CAD build for the part. Positions are in the model's coordinates, mm. Face numbers are marked on the shaded views. A direction names the side the tool comes from. Round coordinates to 2 decimals unless told otherwise and drop trailing zeros. Loops run counter-clockwise (first coordinate to the right, second up) from the corner with the lowest first, then second, coordinate; pieces in that order, holes last. Notation, with made-up numbers: M 78.25,56.25 L 100.25,56.25 A27 cw 100.25,93.25 Z; hole C -32.5,-38.75 d2. An arc over 180 degrees is marked long. Use one line per item in the form item = value.
from build123d import *

# Parameters (mm, degrees)
SKETCH_1_R               = 15
SKETCH_1_R_2             = 11.75
EXTRUDE_1_DEPTH          = 4
SKETCH_2_R               = 11.75
SKETCH_2_R_2             = 9.75
EXTRUDE_2_DEPTH          = 1
FILLET_1_R               = 1
FILLET_2_R               = 1
SKETCH_3_R               = 17.5
SKETCH_3_R_2             = 11.75
EXTRUDE_3_DEPTH          = 0.9
CUT_EXTRUDE_1_DEPTH      = 27.009613607
FILLET_3_R               = 2
FILLET_4_R               = 1
SKETCH_6_R               = 1
CUT_EXTRUDE_2_DEPTH      = 6.5
PATTERN_CIRCULAR_2_COUNT = 3
FILLET_6_R               = 0.5
CHAMFER_1_SIZE           = 0.4
CHAMFER_1_SIZE2          = 2


# Some blends are built 0.0001 mm under size
with BuildPart() as part:
    # 草图1 → 凸台-拉伸1 (new, symmetric)
    with BuildSketch(Plane.XY):
        Circle(SKETCH_1_R)
        Circle(SKETCH_1_R_2, mode=Mode.SUBTRACT)
    extrude(amount=EXTRUDE_1_DEPTH, both=True)

    # 草图2 → 凸台-拉伸2 (add)
    with BuildSketch(Plane(origin=(0, 0, -4), x_dir=(-1, 0, 0), z_dir=(0, 0, -1))):
        Circle(SKETCH_2_R)
        Circle(SKETCH_2_R_2, mode=Mode.SUBTRACT)
    extrude(amount=-EXTRUDE_2_DEPTH)

    # 圆角1
    fillet_1_edges = [part.edges().sort_by_distance(p)[0] for p in [
        (-15, 0, -4),
    ]]
    fillet(fillet_1_edges, radius=FILLET_1_R)

    # 圆角2
    fillet_2_edges = [part.edges().sort_by_distance(p)[0] for p in [
        (9.75, 0, -4),
    ]]
    fillet(fillet_2_edges, radius=FILLET_2_R - 0.0001)  # a hair under: the kernel refuses the full size

    # 草图3 → 凸台-拉伸3 (add)
    with BuildSketch(Plane.XY.offset(4)):
        Circle(SKETCH_3_R)
        with Locations(Location((0, 0, 0), (0, 0, 180))):
            Circle(SKETCH_3_R_2, mode=Mode.SUBTRACT)
    extrude(amount=EXTRUDE_3_DEPTH)

    # 草图4 → 切除-拉伸1 (cut, through all)
    with BuildSketch(Plane(origin=(0, 0, 4), x_dir=(-1, 0, 0), z_dir=(0, 0, -1))):
        with BuildLine():
            Line((-20.056660766, 2), (-15.067846561, 2))
            ThreePointArc((-15.067846561, 2), (-15.2, 0), (-15.067846561, -2))
            Line((-15.067846561, -2), (-20.056660766, -2))
            Line((-20.056660766, -2), (-20.056660766, 2))
        make_face()
    cut_extrude_1 = extrude(amount=-CUT_EXTRUDE_1_DEPTH, mode=Mode.SUBTRACT)

    # 镜向1: 切除-拉伸1 across plane
    add(cut_extrude_1.mirror(Plane(origin=(0, 0, 0), x_dir=(0, 0, 1), z_dir=(1, 0, 0))), mode=Mode.SUBTRACT)

    # 圆角3
    fillet_3_edges = [part.edges().sort_by_distance(p)[0] for p in [
        (-15.067846561, -2, 4.45),
        (-15.067846561, 2, 4.45),
        (15.067846561, -2, 4.45),
        (15.067846561, 2, 4.45),
    ]]
    fillet(fillet_3_edges, radius=FILLET_3_R - 0.0001)  # a hair under: the kernel refuses the full size

    # 圆角4
    fillet_4_edges = [part.edges().sort_by_distance(p)[0] for p in [
        (17.385338651, 2, 4.45),
        (17.385338651, -2, 4.45),
        (-17.385338651, -2, 4.45),
        (-17.385338651, 2, 4.45),
    ]]
    fillet(fillet_4_edges, radius=FILLET_4_R)

    # 草图6 → 切除-拉伸2 (cut)
    with BuildSketch(Plane.XY.offset(4.9)):
        with Locations((0, 14.3)):
            Circle(SKETCH_6_R)
    cut_extrude_2 = extrude(amount=-CUT_EXTRUDE_2_DEPTH, mode=Mode.SUBTRACT)

    # 阵列(圆周)2: 切除-拉伸2 ×3 about axis
    pattern_circular_2_axis = Axis((0, 0, 0), (0, 0, 1))
    for i in range(1, PATTERN_CIRCULAR_2_COUNT):
        add(cut_extrude_2.rotate(pattern_circular_2_axis, i * 360 / PATTERN_CIRCULAR_2_COUNT), mode=Mode.SUBTRACT)

    # 圆角6
    # the kernel refuses this fillet: 0.5 mm, written as the material it takes off along each edge
    with BuildSketch(Plane(origin=(-0.73119563, 14.982167832, -1.6), x_dir=(-0.997111465428935, -0.07595212643607639, 0), z_dir=(0, 0, 1)), Plane(origin=(13.340535761, -6.857849926, -1.6), x_dir=(0.4327792617493751, 0.9014999226842262, 0), z_dir=(0, 0, 1)), Plane(origin=(-12.609340132, -8.124317906, -1.6), x_dir=(0.5643322036795584, -0.8255477962481478, 0), z_dir=(0, 0, 1))) as fillet_6_piece_1:
        with BuildLine():
            CenterArc((0.804059787, 0.49981424), FILLET_6_R, 170.950986261, 100.610876057)
            ThreePointArc((0.310282709, 0.578453903), (0.203956844, 0.26304232), (0, 0))
            ThreePointArc((0, 0), (0.40884396, -0.005572815), (0.817687919, 0))
        make_face()
    extrude(amount=5.6, mode=Mode.SUBTRACT)
    with BuildSketch(Plane(origin=(0.73119563, 14.982167832, -1.6), x_dir=(0.997111465428935, -0.07595212643607635, 0), z_dir=(0, 0, 1)), Plane(origin=(12.609340132, -8.124317906, -1.6), x_dir=(-0.5643322036795624, -0.825547796248145, 0), z_dir=(0, 0, 1)), Plane(origin=(-13.340535761, -6.857849926, -1.6), x_dir=(-0.4327792617493753, 0.9014999226842261, 0), z_dir=(0, 0, 1))) as fillet_6_piece_2:
        with BuildLine():
            CenterArc((0.804059787, -0.49981424), FILLET_6_R, 88.438137682, 100.610876057)
            ThreePointArc((0.310282709, -0.578453903), (0.203956844, -0.26304232), (0, 0))
            ThreePointArc((0, 0), (0.40884396, 0.005572815), (0.817687919, 0))
        make_face()
    extrude(amount=5.6, mode=Mode.SUBTRACT)

    # 倒角1
    chamfer_1_edges = [part.edges().sort_by_distance(p)[0] for p in [
        (11.75, 0, 4.9),
    ]]
    chamfer_1_side = [part.faces().sort_by_distance(p)[0] for p in [
        (15.179125182, 1.457318687, 4.9),
    ]]
    chamfer(chamfer_1_edges, length=CHAMFER_1_SIZE, length2=CHAMFER_1_SIZE2, reference=chamfer_1_side[0])


solid = part.part
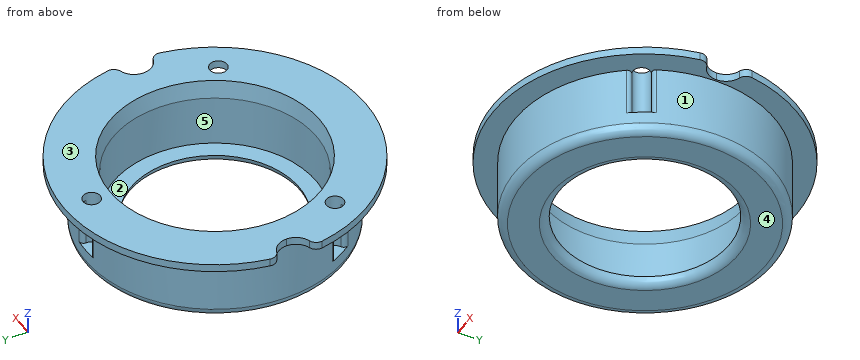
1. Pull direction X, two halves, no side cores. Call the marked faces 1, 2 and 3: +X half, -X half, draft (parallel to the pull), parting line (faces both ways), or undercut.
Completed:
face_1 = parting line
face_2 = undercut
face_3 = draft
2. Cut at A-A on x = 0. State how many separate pieces and enclosed holes the cut face has, and give its area (3 significant figures).
Completed:
separate_pieces = 3
enclosed_holes = 0
area = 53.4 mm2
3. Probe line 1 along Y through (x, z) = (0, 1); line 2 along X through (y, z) = (-0.5, -1.5); line 3 along X through (y, z) = (-8, -2). List the from-to ranges inside material, lowest first. Write a range as from..to.
Completed:
line_1 = -15..-11.75, 11.75..13.3
line_2 = -14.99..-11.74, 11.74..14.99
line_3 = -12.69..-8.61, 8.61..12.69
4. Cut at D-D on z = -2.5. Write the cut outline in (x, y), and give its area (3 significant figures).
Completed:
outline = C 0,0 d30; hole C 0,0 d23.5
area = 273 mm2
5. Drop flat-ended pins along their axis: P1, Ø3, axis at y = -10, z = 3.5, coming from the +X side; P2, Ø1.2, axis at x = 12.38, y = -7.15, coming from the +Z side; P3, Ø1, axis at x = 8.5, z = 0.5, coming from the +Y side. Give the stop position or say it passes through.
Completed:
P1 = 15.25
P2 = -1.6
P3 = 12.69
6. Cut at C-C on z = 3.5. Write the cut outline in (x, y), and give its area (3 significant figures).
Completed:
outline = M -13.69,-6.12 A0.5 ccw -12.95,-6.33 A1 cw long -11.96,-8.05 A0.5 ccw -12.15,-8.8 A15 ccw 12.15,-8.8 A0.5 ccw 11.96,-8.05 A1 cw long 12.95,-6.33 A0.5 ccw 13.69,-6.12 A15 ccw 1.55,14.92 A0.5 ccw 1,14.38 A1 cw long -1,14.38 A0.5 ccw -1.55,14.92 A15 ccw Z; hole C 0,0 d23.74
area = 255 mm2
7. Cut at B-B on z = -0.5. Write the cut outline in (x, y).
Completed:
outline = M -13.69,-6.12 A0.5 ccw -12.95,-6.33 A1 cw long -11.96,-8.05 A0.5 ccw -12.15,-8.8 A15 ccw 12.15,-8.8 A0.5 ccw 11.96,-8.05 A1 cw long 12.95,-6.33 A0.5 ccw 13.69,-6.12 A15 ccw 1.55,14.92 A0.5 ccw 1,14.38 A1 cw long -1,14.38 A0.5 ccw -1.55,14.92 A15 ccw Z; hole C 0,0 d23.5
8. Tool access for the marked faces 4 and 5: list every direction of +Z, -Z, +X, -X, +Y, -Y with a clear straight run to the whole face (end or side of a thin tool).
Completed:
face_4 = -Z, +X, -X, +Y, -Y
face_5 = +Z
